Here's how the part is built. I have some questions about the finished solid (model axes, mm). Face numbers are marked on the shaded views. A direction names the side the tool comes from. Give positions to 0.01 mm unless a question says otherwise; leave off trailing zeros. Loops run counter-clockwise (first coordinate to the right, second up) from the corner with the lowest first, then second, coordinate; pieces in that order, holes last. Notation, with made-up numbers: (51, -24.75) - (99, -24.75) arc R25 cw to (99, -6.75) - close; hole circle Ø2 at (68, -10). An arc over 180 degrees is marked (long way). Put each result on its own line as item: value. Start each with the question number.
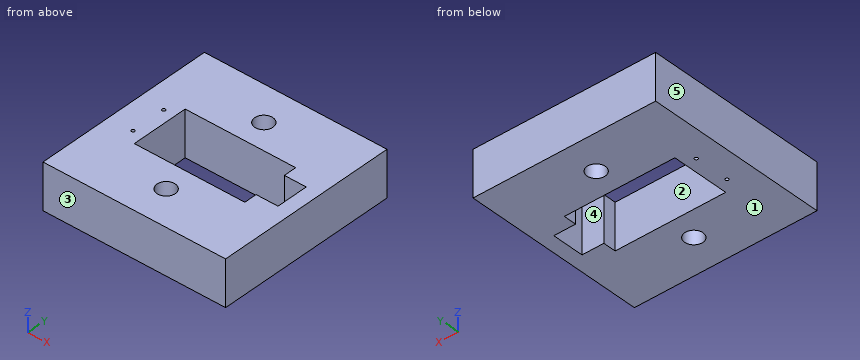
from build123d import *

# Parameters (mm, degrees)
F0_W     = 40
F0_H     = 40
F0_R     = 0.35
F0_R_2   = 2
F1_DEPTH = 10


with BuildPart() as f1:
    # F0 (on Top) → F1 (new body)
    with BuildSketch(Plane.XY):
        with Locations((20, 20)):
            Rectangle(F0_W, F0_H)
        with Locations((5.4065, 16.2)):
            Circle(F0_R, mode=Mode.SUBTRACT)
        with Locations((20, 7.9)):
            Circle(F0_R_2, mode=Mode.SUBTRACT)
        with Locations((5.4065, 23.8)):
            Circle(F0_R, mode=Mode.SUBTRACT)
        Polygon((7.8935, 13.7), (7.8935, 26.3), (32.1065, 26.3), (32.1065, 23.5), (36.8935, 23.5), (36.8935, 16.5), (32.1065, 16.5), (32.1065, 13.7), align=None, mode=Mode.SUBTRACT)
        with Locations((20, 32.1)):
            Circle(F0_R_2, mode=Mode.SUBTRACT)
    extrude(amount=F1_DEPTH)


solid = f1.part
1) I need wall thicknesses on line 1 (X direction, y = 23.8, z = 3); line 2 (Y direction, x = 20, z = 7); line 3 (X direction, y = 17, z = 7). Which ranges of each line are inside material? Lowest first, please.
2) Suppose I cut it at B-B on x = 15.5. Please give me the cut outline in (y, z).
3) Suppose I cut it at A-A on z = 5.75. Please give me the cut outline in (x, y), plus the area to 3 significant figures.
4) Thinking about a two-plate mould opening in Y: for the marked faces 1, 2 and 3, which applies, pulls with the +Y half, pulls with the -Y half, needs draft (parallel to the pull), parting line crosses it, or undercut?
5) Which directions (+Z, -Z, +X, -X, +Y, -Y) give clear straight access to the entire face, cutting with the end or side of a thin tool? Please do the marked faces 4 and 5.
6) I'm going to push a flat-ended pin straight in: P1, Ø3, axis at y = 7, z = 3.5, coming from the -X side. Where does the tip first touch, or does it pass through?
7) Suppose I cut it at C-C on y = 20. Please give me the cut outline in (x, z), plus the area to 3 significant figures.
Ans:
1. line 1: x = 0 to 5.06, 5.76 to 7.89, 32.11 to 40
1. line 2: y = 0 to 5.9, 9.9 to 13.7, 26.3 to 30.1, 34.1 to 40
1. line 3: x = 0 to 7.89, 36.89 to 40
2. outline: (0, 0) - (13.7, 0) - (13.7, 10) - (0, 10) - close; (26.3, 0) - (40, 0) - (40, 10) - (26.3, 10) - close
3. outline: (0, 0) - (40, 0) - (40, 40) - (0, 40) - close; hole circle Ø0.7 at (5.41, 16.2); hole circle Ø0.7 at (5.41, 23.8); hole (7.89, 13.7) - (32.11, 13.7) - (32.11, 16.5) - (36.89, 16.5) - (36.89, 23.5) - (32.11, 23.5) - (32.11, 26.3) - (7.89, 26.3) - close; hole circle Ø4 at (20, 7.9); hole circle Ø4 at (20, 32.1)
3. area: 1,240 mm²
4. face 1: needs draft
4. face 2: undercut
4. face 3: pulls with the -Y half
5. face 4: +Z, -Z
5. face 5: +Z, -Z, -X, +Y, -Y
6. P1: stops at x = 0
7. outline: (0, 0) - (7.89, 0) - (7.89, 10) - (0, 10) - close; (36.89, 0) - (40, 0) - (40, 10) - (36.89, 10) - close
7. area: 110 mm²
